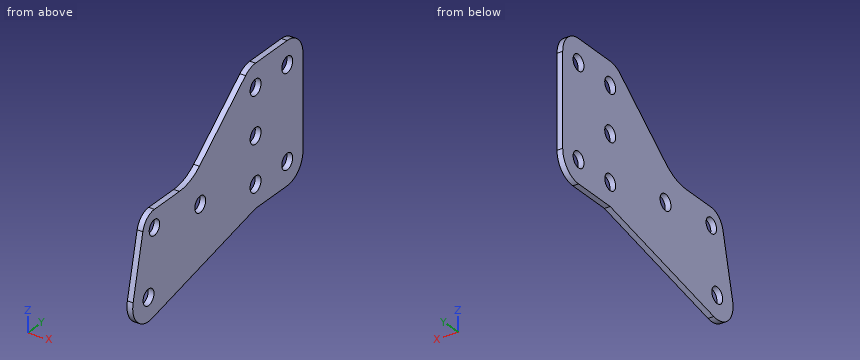
Autodesk Inventor part; units mm, degrees
ref_plane "YZ Plane" through (0, 0, 0) normal (1, 0, 0) x (0, 1, 0)
ref_plane "XZ Plane" through (0, 0, 0) normal (0, 1, 0) x (-1, 0, 0)
ref_plane "XY Plane" through (0, 0, 0) normal (0, 0, 1) x (1, 0, 0)
sketch "maiin" plane through (0, 0, 0) normal (0, 0, 1) x (1, 0, 0)
  circle A0 centre (-6.5018, 3.4753) radius 2.1844
  line L0 (-6.8203, 13.6107) -> (11.7059, 28.671)
  circle A1 centre (-27.2482, -11.1789) radius 2.1844
  arc A2 (-33.4335, -9.7418) -> (-25.8521, -17.3735) centre (-27.2482, -11.1789) ccw
  line L1 (34.75, -1.6563) -> (34.75, 23.7437)
  line L2 (15.7114, 30.0937) -> (28.4, 30.0937)
  circle A3 centre (28.4114, 23.7437) radius 2.1844
  circle A4 centre (28.4, -1.6563) radius 2.1844
  circle A5 centre (15.7114, 23.7437) radius 2.1844
  circle A6 centre (15.7, -1.6563) radius 2.1844
  arc A7 (34.75, 23.7437) -> (28.4, 30.0937) centre (28.4, 23.7437) ccw
  arc A8 (15.7114, 30.0937) -> (11.7059, 28.671) centre (15.7114, 23.7437) ccw
  arc A9 (28.4, -8.0063) -> (34.75, -1.6563) centre (28.4, -1.6563) ccw
  line L3 (28.4, -8.0063) -> (15.7114, -8.0063)
  line L4 (15.7114, -8.0063) -> (-25.8521, -17.3735)
  circle A10 centre (-24.886, 6.0028) radius 2.0955
  arc A11 (-24.886, 10.7653) -> (-29.5249, 7.0806) centre (-24.886, 6.0028) ccw
  line L5 (-33.4335, -9.7418) -> (-29.5249, 7.0806)
  line L6 (-14.8313, 10.7653) -> (-24.886, 10.7653)
  arc A12 (-14.8313, 10.7653) -> (-6.8203, 13.6107) centre (-14.8313, 23.4653) ccw
  point P0 (10.0881, 4.3711)
  point P1 (32.8902, 28.2338)
  dimension "d0" = 12.7
  dimension "d6" = 4.3688
  dimension "d9" = 12.7
  dimension "d10" = 25.4
  dimension "d11" = 12.7
  dimension "d12" = 25.4
  dimension "d14" = 4.191
  dimension "d15" = 9.525
  dimension "d16" = 12.7
sketch "Sketch1" plane through (0, 0, 0) normal (1, 0, 0) x (0, 1, 0)
  circle A0 centre (-12.7, -12.7) radius 2.1844
  circle A1 centre (-34.9132, -20.2684) radius 2.1844
  line L0 (-35.2318, -10.133) -> (-16.7055, 4.9273)
  circle A2 centre (-55.6596, -34.9226) radius 2.1844
  arc A3 (-61.8449, -33.4855) -> (-54.2635, -41.1172) centre (-55.6596, -34.9226) ccw
  line L1 (6.3386, -25.4) -> (6.3386, 0)
  line L2 (-12.7, 6.35) -> (-0.0114, 6.35)
  circle A4 centre (0, 0) radius 2.1844
  circle A5 centre (-0.0114, -25.4) radius 2.1844
  circle A6 centre (-12.7, 0) radius 2.1844
  circle A7 centre (-12.7114, -25.4) radius 2.1844
  arc A8 (6.3386, 0) -> (-0.0114, 6.35) centre (-0.0114, 0) ccw
  arc A9 (-12.7, 6.35) -> (-16.7055, 4.9273) centre (-12.7, 0) ccw
  arc A10 (-0.0114, -31.75) -> (6.3386, -25.4) centre (-0.0114, -25.4) ccw
  line L3 (-0.0114, -31.75) -> (-12.7, -31.75)
  line L4 (-12.7, -31.75) -> (-54.2635, -41.1172)
  circle A11 centre (-53.2974, -17.7408) radius 2.0955
  arc A12 (-53.2974, -12.9783) -> (-57.9364, -16.663) centre (-53.2974, -17.7408) ccw
  line L5 (-61.8449, -33.4855) -> (-57.9364, -16.663)
  line L6 (-43.2428, -12.9783) -> (-53.2974, -12.9783)
  arc A13 (-43.2428, -12.9783) -> (-35.2318, -10.133) centre (-43.2428, -0.2783) ccw
  dimension "d17" = 4.3688
extrude "Extrusion1" add sketch "Sketch1" along normal blind 1.5875
properties part number "Angle Brace Gusset" material "Acetal Resin, White"
Model file for the job. Use its own axes, mm. Give positions to 0.01 mm unless a question says otherwise; leave off trailing zeros. Loops run counter-clockwise (first coordinate to the right, second up) from the corner with the lowest first, then second, coordinate; pieces in that order, holes last. Notation, with made-up numbers: (69, 23) -> (115, 23) arc R33 ccw to (115, 53) -> close; hole circle Ø11 at (-13, -13.75). An arc over 180 degrees is marked (long way). Use a Markdown table: item, result. Add a question column.
(1) Slice it at C-C on y = -46. List the corners of the cut face in (x, z), and give its area (3 significant figures).
(2) Slice it at A-A on y = -11.5. List the corners of the cut face in (x, z), and give its area (3 significant figures).
(3) Slice it at B-B on x = 0.9. Give the number of separate pieces and of enclosed holes in the cut face, and give its area (3 significant figures).
(4) Wall check: line 1 along Z through (x, y) = (0.7, -12.7); line 2 along Z through (x, y) = (1, 0); line 3 along Y through (x, z) = (1.55, 1.5). Give the ranges that are in metal, low to high.
Filled sheet:
| question | item | result |
|---|---|---|
| 1 | outline | (0, -39.25) -> (1.59, -39.25) -> (1.59, -12.98) -> (0, -12.98) -> close |
| 1 | area | 41.7 mm2 |
| 2 | outline | (0, -31.75) -> (1.59, -31.75) -> (1.59, -27.22) -> (0, -27.22) -> close; (0, -23.58) -> (1.59, -23.58) -> (1.59, -14.53) -> (0, -14.53) -> close; (0, -10.87) -> (1.59, -10.87) -> (1.59, -1.83) -> (0, -1.83) -> close; (0, 1.83) -> (1.59, 1.83) -> (1.59, 6.35) -> (0, 6.35) -> close |
| 2 | area | 43.1 mm2 |
| 3 | separate pieces | 1 |
| 3 | enclosed holes | 8 |
| 3 | area | 1,990 mm2 |
| 4 | line 1 | -31.75 to -27.58, -23.22 to -14.88, -10.52 to -2.18, 2.18 to 6.35 |
| 4 | line 2 | -31.75 to -27.58, -23.22 to -2.18, 2.18 to 6.35 |
| 4 | line 3 | -20.92 to -14.29, -11.11 to -1.59, 1.59 to 6.16 |
